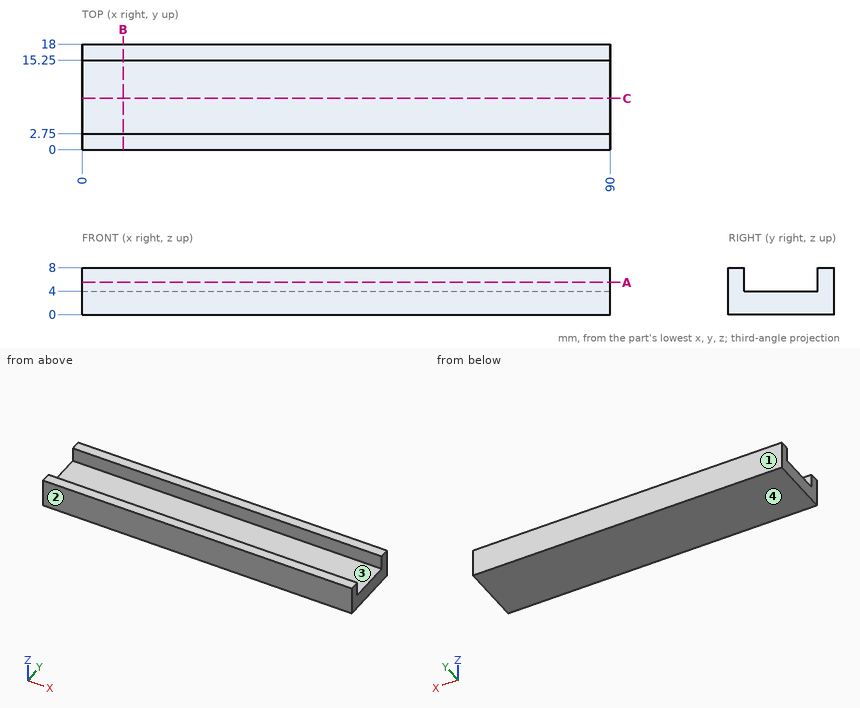
Can you work these out from the drawing? Everything is in mm from the part's minimum corner. Round coordinates to 2 decimals unless told otherwise and drop trailing zeros. Loops run counter-clockwise (first coordinate to the right, second up) from the corner with the lowest first, then second, coordinate; pieces in that order, holes last. Notation, with made-up numbers: (-3, -32) - (28, -32) arc R16 cw to (28, -20) - close; hole circle Ø6 at (41, -22). An arc over 180 degrees is marked (long way). Answer in a Markdown table with one row per item. Add a question column.
(1) I need wall thicknesses on line 1 along Y through (x, z) = (74, 7.25); line 2 along Z through (x, y) = (21, 13). Which ranges of each line are inside material? Lowest first, please.
(2) If we section it at A-A (z = 5.5): Please give me the cut outline in (x, y).
(3) If we section it at C-C (y = 8.75): Please give me the cut outline in (x, z), plus the area to 3 significant figures.
(4) If we mould it in two halves opening along Y, with no side actions, what happens to the marked faces 1, 2, 3 and 4? For each: pulls with the +Y half, pulls with the -Y half, needs draft (parallel to the pull), parting line crosses it, or undercut.
(5) If we section it at B-B (x = 7): Please give me the cut outline in (y, z), plus the area to 3 significant figures.
(6) I'm going to push a flat-ended pin straight in: pin 1 (4 mm diameter, centred on x = 45, y = 8, fed in from +Z). Where does the tip first touch, or does it pass through?
Model answer:
| question | item | result |
|---|---|---|
| 1 | line 1 | y = 0 to 2.75, 15.25 to 18 |
| 1 | line 2 | z = 0 to 4 |
| 2 | outline | (0, 0) - (90, 0) - (90, 2.75) - (0, 2.75) - close; (0, 15.25) - (90, 15.25) - (90, 18) - (0, 18) - close |
| 3 | outline | (0, 0) - (90, 0) - (90, 4) - (0, 4) - close |
| 3 | area | 360 mm² |
| 4 | face 1 | pulls with the +Y half |
| 4 | face 2 | pulls with the -Y half |
| 4 | face 3 | undercut |
| 4 | face 4 | needs draft |
| 5 | outline | (0, 0) - (18, 0) - (18, 8) - (15.25, 8) - (15.25, 4) - (2.75, 4) - (2.75, 8) - (0, 8) - close |
| 5 | area | 94.0 mm² |
| 6 | pin 1 | stops at z = 4 |
